Autodesk Inventor part; units mm, degrees
ref_plane "YZ Plane" through (0, 0, 0) normal (1, 0, 0) x (0, 1, 0)
ref_plane "XZ Plane" through (0, 0, 0) normal (0, 1, 0) x (-1, 0, 0)
ref_plane "XY Plane" through (0, 0, 0) normal (0, 0, 1) x (1, 0, 0)
sketch "Sketch1" plane through (0, 0, 0) normal (0, 0, 1) x (1, 0, 0)
  line L0 (-1066.8, 304.8) -> (1066.8, 304.8)
  line L1 (1066.8, 304.8) -> (1066.8, -304.8)
  line L2 (1066.8, -304.8) -> (-1066.8, -304.8)
  line L3 (-1066.8, -304.8) -> (-1066.8, 304.8)
  point P0 (0, 0)
  point P1 (1066.8, 0)
  point P2 (0, 304.8)
  dimension "d0" = 2133.6
  dimension "d1" = 609.6
extrude "Extrusion1" add sketch "Sketch1" along normal mid plane 25.4
sketch "Sketch2" plane through (0, 0, 12.7) normal (0, 0, 1) x (1, 0, 0)
  circle A0 centre (736.6, 241.3) radius 38.1
  line L0 (1066.8, -304.8) -> (1066.8, 304.8)
  line L1 (-1066.8, 304.8) -> (1066.8, 304.8)
  circle A1 centre (736.6, -266.7) radius 38.1
  line L2 (-1066.8, -304.8) -> (1066.8, -304.8)
  circle A2 centre (-787.4, 266.7) radius 38.1
  circle A3 centre (-736.6, -266.7) radius 38.1
  line L3 (-1066.8, 304.8) -> (-1066.8, -304.8)
  point P0 (0, 0)
  dimension "d4" = 330.2
  dimension "d5" = 63.5
  dimension "d6" = 76.2
  dimension "d7" = 76.2
  dimension "d8" = 330.2
  dimension "d9" = 38.1
  dimension "d10" = 76.2
  dimension "d11" = 76.2
  dimension "d12" = 279.4
  dimension "d13" = 330.2
  dimension "d14" = 38.1
  dimension "d15" = 38.1
extrude "Extrusion2" add sketch "Sketch2" along normal blind 101.6 contours A0 | A2 | A3 | A1
sketch "Sketch3" plane through (0, 0, 12.7) normal (0, 0, 1) x (1, 0, 0)
  line L0 (-1066.8, -304.8) -> (-1066.8, 304.8)
  line L1 (1066.8, -304.8) -> (-1066.8, -304.8)
  line L2 (-1066.8, 304.8) -> (-1041.4, 304.8)
  line L3 (-1041.4, 304.8) -> (-1041.4, -304.8)
  line L4 (-1041.4, -304.8) -> (-1066.8, -304.8)
  line L5 (-1066.8, -304.8) -> (-1066.8, 304.8)
  line L6 (1066.8, 304.8) -> (1041.4, 304.8)
  line L7 (1041.4, 304.8) -> (1041.4, -304.8)
  line L8 (1041.4, -304.8) -> (1066.8, -304.8)
  line L9 (1066.8, -304.8) -> (1066.8, 304.8)
  point P0 (0, 0)
  dimension "d18" = 25.4
  dimension "d19" = 25.4
extrude "Extrusion3" add sketch "Sketch3" along normal blind 203.2
sketch "Sketch5" plane through (0, 0, 0) normal (0, 1, 0) x (-1, 0, 0)
  line L0 (-1041.4, 12.7) -> (787.4, 12.7)
  point P0 (0, 0)
sketch "Sketch6" plane through (0, 0, 12.7) normal (0, 0, 1) x (1, 0, 0)
  line L0 (-1041.4, 304.8) -> (-1041.4, -304.8)
  line L1 (-1041.4, 304.8) -> (-965.2, 304.8)
  line L2 (-965.2, 304.8) -> (-965.2, 177.8)
  line L3 (-965.2, 177.8) -> (-1041.4, 177.8)
  line L4 (-1041.4, 177.8) -> (-1041.4, 304.8)
  line L5 (-1041.4, -304.8) -> (-965.2, -304.8)
  line L6 (-965.2, -304.8) -> (-965.2, -177.8)
  line L7 (-965.2, -177.8) -> (-1041.4, -177.8)
  line L8 (-1041.4, -177.8) -> (-1041.4, -304.8)
  point P0 (0, 0)
  dimension "d30" = 76.2
  dimension "d31" = 127
  dimension "d32" = 127
  dimension "d33" = 76.2
extrude "Extrusion5" add sketch "Sketch6" along normal blind 203.2
mirror "Mirror1" about plane through (0, 0, 0) normal (1, 0, 0) of "Extrusion5"
fillet "Fillet1" radius 50.8 4 edges at (-965.2, 177.8, 114.3) (965.2, 177.8, 114.3) (965.2, -177.8, 114.3) (-965.2, -177.8, 114.3)
sketch "Sketch14" plane through (0, 0, -12.7) normal (0, 0, -1) x (-1, 0, 0)
  line L0 (-1066.8, 304.8) -> (1066.8, 304.8)
  line L1 (1066.8, 304.8) -> (1066.8, 330.2)
  line L2 (1066.8, 330.2) -> (-1066.8, 330.2)
  line L3 (-1066.8, 330.2) -> (-1066.8, 304.8)
  line L4 (1066.8, -304.8) -> (-1066.8, -304.8)
  line L5 (-1066.8, -304.8) -> (-1066.8, -330.2)
  line L6 (-1066.8, -330.2) -> (1066.8, -330.2)
  line L7 (1066.8, -330.2) -> (1066.8, -304.8)
  point P0 (0, 0)
  dimension "d62" = 25.4
  dimension "d63" = 25.4
extrude "Extrusion11" add sketch "Sketch14" against normal blind 228.6
sketch "Sketch15" plane through (-1066.8, 330.2, -12.7) normal (0, 1, 0) x (1, 0, 0)
  line L0 (2133.6, 0) -> (2133.6, -228.6)
  line L1 (2133.6, -228.6) -> (2133.6, -254)
  line L2 (2133.6, -254) -> (1879.6, -254)
  line L3 (1879.6, -254) -> (1371.6, -457.2)
  line L4 (1371.6, -457.2) -> (762, -457.2)
  line L5 (762, -457.2) -> (254, -254)
  line L6 (254, -254) -> (0, -254)
  line L7 (0, -254) -> (0, -228.6)
  line L8 (0, -228.6) -> (2133.6, -228.6)
  point P0 (1066.8, -12.7)
  dimension "d66" = 254
  dimension "d67" = 508
  dimension "d68" = 609.6
  dimension "d69" = 508
  dimension "d70" = 254
  dimension "d71" = 228.6
  dimension "d72" = 25.4
  dimension "d73" = 25.4
extrude "Extrusion12" add sketch "Sketch15" against normal blind 25.4
mirror "Mirror4" about plane through (0, 0, 0) normal (0, 1, 0) of "Extrusion12"
sketch "Sketch16" plane through (0, 0, -12.7) normal (0, 0, -1) x (-1, 0, 0)
  line L0 (-457.2, -177.8) -> (-457.2, -76.2)
  line L1 (-355.6, -177.8) -> (-355.6, -76.2)
  arc A0 (-355.6, -76.2) -> (-457.2, -76.2) centre (-406.4, -76.2) ccw
  arc A1 (-457.2, -177.8) -> (-355.6, -177.8) centre (-406.4, -177.8) ccw
  line L2 (-1066.8, 330.2) -> (-1066.8, -330.2)
  line L3 (-1066.8, -330.2) -> (1066.8, -330.2)
  point P0 (0, 0)
  dimension "d76" = 101.6
  dimension "d77" = 609.6
  dimension "d78" = 152.4
  dimension "d79" = 101.6
extrude "Extrusion13" cut sketch "Sketch16" against normal blind 25.4
sketch "Sketch20" plane through (0, 0, 12.7) normal (0, 0, 1) x (1, 0, 0)
  line L0 (-965.2, 304.8) -> (-1066.8, 304.8)
  line L1 (-1041.4, 304.8) -> (-749.3, 304.8)
  line L2 (-749.3, 304.8) -> (-749.3, 228.6)
  line L3 (-749.3, 228.6) -> (-1041.4, 228.6)
  line L4 (-1041.4, 228.6) -> (-1041.4, 304.8)
  line L5 (-965.2, -304.8) -> (-1028.7, -304.8)
  line L6 (-1016, -304.8) -> (-698.5, -304.8)
  line L7 (-698.5, -304.8) -> (-698.5, -228.6)
  line L8 (-698.5, -228.6) -> (-1016, -228.6)
  line L9 (-1016, -228.6) -> (-1016, -304.8)
  point P0 (0, 0)
extrude "Extrusion16" add sketch "Sketch20" along normal blind 101.6
mirror "Mirror5" about plane through (0, 0, 0) normal (1, 0, 0) of "Extrusion16"
sketch "Sketch21" plane through (0, 0, 12.7) normal (0, 0, 1) x (1, 0, 0)
  line L0 (812.8, 304.8) -> (304.8, 304.8)
  line L1 (681.4009, 304.8) -> (770.3009, 304.8)
  line L2 (770.3009, 304.8) -> (770.3009, 177.8)
  line L3 (770.3009, 177.8) -> (681.4009, 177.8)
  line L4 (681.4009, 177.8) -> (681.4009, 304.8)
  point P0 (0, 0)
  dimension "d91" = 127
  dimension "d92" = 88.9
extrude "Extrusion17" add sketch "Sketch21" along normal blind 101.6
sketch "Sketch22" plane through (0, 0, 12.7) normal (0, 0, 1) x (1, 0, 0)
  line L0 (-812.8, 304.8) -> (-1066.8, 304.8)
  line L1 (-812.8, -304.8) -> (-1066.8, -304.8)
  line L2 (-1041.4, 304.8) -> (-927.1, 304.8)
  line L3 (-927.1, 304.8) -> (-927.1, -304.8)
  line L4 (-927.1, -304.8) -> (-1041.4, -304.8)
  line L5 (-1041.4, -304.8) -> (-1041.4, 304.8)
  line L6 (-1041.4, -177.8) -> (-1041.4, 177.8)
  point P0 (0, 0)
  dimension "d97" = 114.3
  dimension "d98" = 0
extrude "Extrusion18" add sketch "Sketch22" along normal blind 101.6
mirror "Mirror7" about plane through (0, 0, 0) normal (1, 0, 0) of "Extrusion18"
sketch "Sketch23" plane through (-1066.8, -330.2, -12.7) normal (0, -1, 0) x (1, 0, 0)
  circle A0 centre (76.2, 76.2) radius 38.1
  line L0 (0, 0) -> (0, 254)
  line L1 (2133.6, 0) -> (0, 0)
  point P0 (1066.8, 12.7)
  dimension "d101" = 76.2
  dimension "d102" = 76.2
  dimension "d103" = 76.2
extrude "Extrusion19" cut sketch "Sketch23" against normal blind 152.4
mirror "Mirror8" about plane through (0, 0, 0) normal (1, 0, 0) of "Extrusion19"
properties part number "Cam_support2"
Read the model definition and answer for the solid it produces. Units are mm, in the model's axes. A direction names the side the tool comes from. Give positions to 0.01 mm unless a question says otherwise; leave off trailing zeros. Write each loop counter-clockwise with the first axis right and the second up, starting at its lowest first coordinate (ties: lowest second). Pieces come first, ordered by that corner, then holes. Notation, with made-up numbers: (-38.5, -5.5) -> (-2.5, -5.5) arc R17 ccw to (-2.5, 14.5) -> close; hole circle Ø2 at (49, -25.75). An arc over 180 degrees is marked (long way). Answer as a JSON object with one key per item and string values.
1) Section A-A on z = 307.5 is taken. Write down the section's boundary in (x, y), then the cut area to 3 significant figures.
Findings below:
{"outline": "(-647.3, -330.2) -> (647.3, -330.2) -> (647.3, -304.8) -> (-647.3, -304.8) -> close; (-647.3, 304.8) -> (647.3, 304.8) -> (647.3, 330.2) -> (-647.3, 330.2) -> close", "area": "65,800 mm^2"}
2) Section D-D on z = 63.5 is taken. Write down the section's boundary in (x, y), then the cut area to 3 significant figures.
Findings below:
{"outline": "(-1066.8, -330.2) -> (-1028.7, -330.2) -> (-1028.7, -177.8) -> (-952.5, -177.8) -> (-952.5, -330.2) -> (952.5, -330.2) -> (952.5, -177.8) -> (1028.7, -177.8) -> (1028.7, -330.2) -> (1066.8, -330.2) -> (1066.8, 330.2) -> (-1066.8, 330.2) -> close; hole (-927.1, -228.6) -> (-698.5, -228.6) -> (-698.5, -304.8) -> (698.5, -304.8) -> (698.5, -228.6) -> (927.1, -228.6) -> (927.1, 228.6) -> (772.52, 228.6) arc R38.1 cw to (770.3, 223.53) -> (770.3, 177.8) -> (681.4, 177.8) -> (681.4, 304.8) -> (-749.3, 304.8) -> (-749.3, 228.6) -> (-927.1, 228.6) -> close", "area": "327,000 mm^2"}
3) A tool of negligible diameter and unlimited length cuts with its end or side. For faces 1 (the flat face through (-562.356, -317.678, 341.478)), 2 (the flat face through (-991, -177.8, 64)), 3 (the flat face through (681.401, 240, 63)), from which of +Z, -Z, +X, -X, +Y, -Y can it reach the whole face along a straight path? Write none if from no direction.
Findings below:
{"face 1": "+Z, -X, +Y, -Y", "face 2": "-Y", "face 3": "+Z"}
4) Straight lines are drawn through the part: probe 1 along Y at (x, z) = (-658, 131); probe 2 along X at (y, z) = (-292, 63); probe 3 along Y at (x, z) = (777, 57). For each, find the intervals that lie inside material, in ascending order. Write a range as from..to.
Findings below:
{"probe 1": "y = -330.2..-304.8, 304.8..330.2", "probe 2": "x = -1066.8..-1028.7, -952.5..-698.5, 698.5..952.5, 1028.7..1066.8", "probe 3": "y = -330.2..-228.6, 228.6..330.2"}
5) Flat-ended cylindrical pins translate along their axes: pin 1 Ø4 at (x, y) = (-318.5, -34.5) entering from +Z; pin 2 Ø12.5 at (x, y) = (-904.5, -316.5) entering from +Z; pin 3 Ø23 at (x, z) = (994, 61.5) entering from -Y. Find the tip coordinate at first contact, or state that the pin passes through.
Findings below:
{"pin 1": "stops at z = 12.7", "pin 2": "stops at z = 241.3", "pin 3": "stops at y = -177.8"}
6) Section B-B on y = -126 is taken. Write down the section's boundary in (x, z), then the cut area to 3 significant figures.
Findings below:
{"outline": "(-1066.8, -12.7) -> (355.6, -12.7) -> (355.6, 12.7) -> (-927.1, 12.7) -> (-927.1, 114.3) -> (-1041.4, 114.3) -> (-1041.4, 215.9) -> (-1066.8, 215.9) -> close; (457.2, -12.7) -> (1066.8, -12.7) -> (1066.8, 215.9) -> (1041.4, 215.9) -> (1041.4, 114.3) -> (927.1, 114.3) -> (927.1, 12.7) -> (457.2, 12.7) -> close", "area": "85,200 mm^2"}
7) Section C-C on x = 406.4 is taken. Write down the section's boundary in (y, z).
Findings below:
{"outline": "(-330.2, -12.7) -> (-228.6, -12.7) -> (-228.6, 12.7) -> (-304.8, 12.7) -> (-304.8, 403.86) -> (-330.2, 403.86) -> close; (-25.4, -12.7) -> (330.2, -12.7) -> (330.2, 403.86) -> (304.8, 403.86) -> (304.8, 12.7) -> (-25.4, 12.7) -> close"}
8) For a pull along Z with two mould halves and no side action, classify faces 4 (the cylindrical face through (-954.26, -255.07, 74.94)), 5 (the flat face through (939, 4, 114.3)), 6 (the cylindrical face through (980.476, -192.286, 165.811)) as pulls with the +Z half, pulls with the -Z half, needs draft (parallel to the pull), parting line crosses it, or undercut.
Findings below:
{"face 4": "undercut", "face 5": "pulls with the +Z half", "face 6": "needs draft"}
